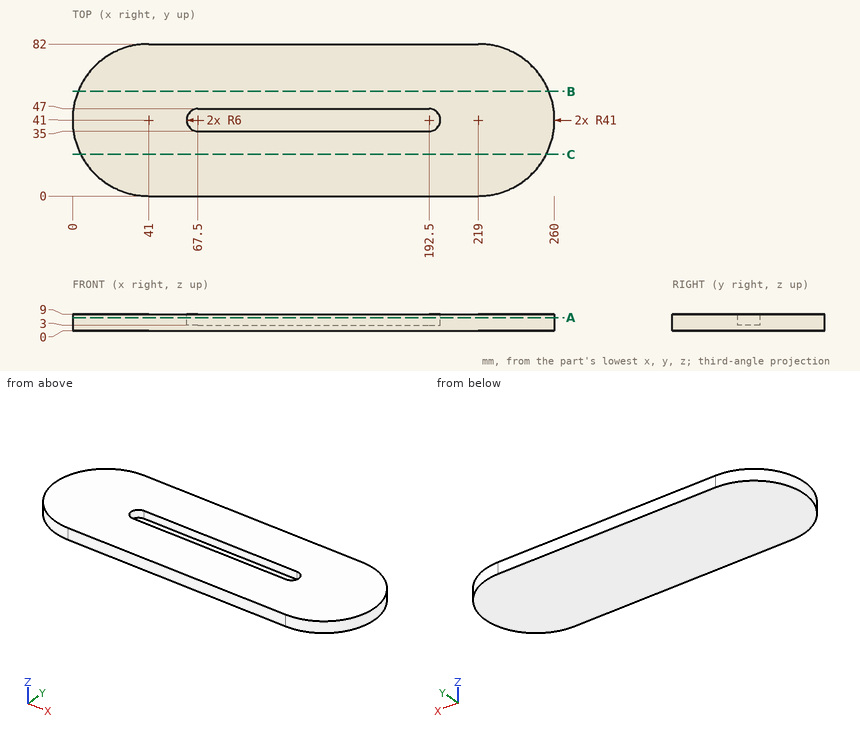
Source: three-view drawing plus pictorial views. Frame: mm from the lowest corner of the part. Coordinates: 2 decimals unless noted, no trailing zeros. Loops run counter-clockwise (first coordinate to the right, second up) from the corner with the lowest first, then second, coordinate; pieces in that order, holes last. Notation, with made-up numbers: M -14.75,-39.75 L 33.25,-39.75 A19 cw 33.25,-27.75 Z; hole C 85,36.25 d9. An arc over 180 degrees is marked long. Use CSV: the item, a comma, the result in double quotes.
(1) Cut plane C-C on y = 22.5. Return loops of the section in (x, z), and give its area (3 significant figures).
Answers follow:
outline,"M 4.41,0 L 255.59,0 L 255.59,9 L 4.41,9 Z"
area,"2,260 mm²"
(2) Contact query for flat-ended pins moving along their axis: pin 1 (6 mm diameter, centred on x = 123, y = 41.5, fed in from +Z); pin 2 (3 mm diameter, centred on y = 52, z = 3, fed in from +X); pin 3 (3 mm diameter, centred on y = 58, z = 2, fed in from +X). Output: stop coordinate, or through.
Answers follow:
pin 1,"z = 3"
pin 2,"x = 258.88"
pin 3,"x = 256.96"
(3) Cut plane A-A on z = 7. Return loops of the section in (x, y), and give its area (3 significant figures).
Answers follow:
outline,"M 41,0 L 219,0 A41 ccw 219,82 L 41,82 A41 ccw Z; hole M 67.5,35 L 192.5,35 A6 ccw 192.5,47 L 67.5,47 A6 ccw Z"
area,"18,300 mm²"
(4) Cut plane B-B on y = 56.5. Return loops of the section in (x, z), and give its area (3 significant figures).
Answers follow:
outline,"M 3.04,0 L 256.96,0 L 256.96,9 L 3.04,9 Z"
area,"2,290 mm²"
(5) Line query: line 1 (Y direction, x = 78, z = 4.5); line 2 (X direction, y = 40.5, z = 4.25); line 3 (Z direction, x = 118.5, y = 43). Output: solid intervals per line, ascending. Write a range as [from, to].
Answers follow:
line 1,"[0, 35], [47, 82]"
line 2,"[0, 61.52], [198.48, 260]"
line 3,"[0, 3]"
